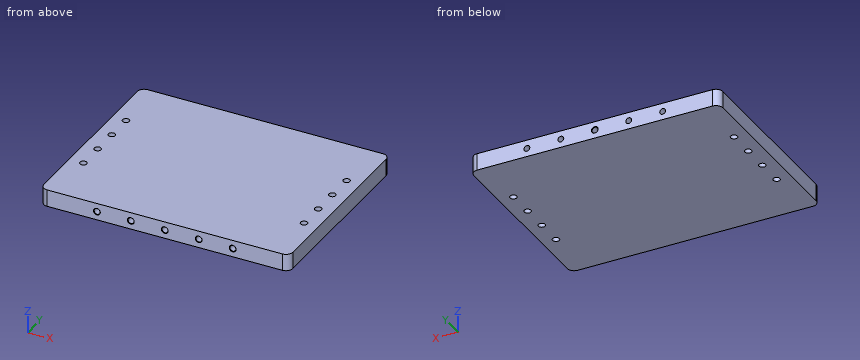
from build123d import *

# Parameters (mm, degrees)
SKETCH_1_R          = 1.5
EXTRUDE_1_DEPTH     = 7.5
SKETCH_2_R          = 1.3
CUT_EXTRUDE_1_DEPTH = 7.5
CUT_EXTRUDE_START   = -7.5
SKETCH_3_R          = 1.3
CUT_EXTRUDE_2_DEPTH = 7.5
CHAMFER_1_SIZE      = 0.2
CHAMFER_2_SIZE      = 0.2


with BuildPart() as part:
    # Sketch 1 → Extrude 1 (new body)
    with BuildSketch(Plane.XY):
        with BuildLine():
            Line((-52, -42.5), (52, -42.5))
            ThreePointArc((52, -42.5), (54.121320344, -41.621320344), (55, -39.5))
            Line((55, -39.5), (55, 39.5))
            ThreePointArc((55, 39.5), (54.121320344, 41.621320344), (52, 42.5))
            Line((52, 42.5), (-52, 42.5))
            ThreePointArc((-52, 42.5), (-54.121320344, 41.621320344), (-55, 39.5))
            Line((-55, 39.5), (-55, -39.5))
            ThreePointArc((-55, -39.5), (-54.121320344, -41.621320344), (-52, -42.5))
        make_face()
        with Locations((48.75, 18)):
            Circle(SKETCH_1_R, mode=Mode.SUBTRACT)
        with Locations((48.75, 6)):
            Circle(SKETCH_1_R, mode=Mode.SUBTRACT)
        with Locations((48.75, -6)):
            Circle(SKETCH_1_R, mode=Mode.SUBTRACT)
        with Locations((48.75, -18)):
            Circle(SKETCH_1_R, mode=Mode.SUBTRACT)
        with Locations((-48.75, -18)):
            Circle(SKETCH_1_R, mode=Mode.SUBTRACT)
        with Locations((-48.75, -6)):
            Circle(SKETCH_1_R, mode=Mode.SUBTRACT)
        with Locations((-48.75, 6)):
            Circle(SKETCH_1_R, mode=Mode.SUBTRACT)
        with Locations((-48.75, 18)):
            Circle(SKETCH_1_R, mode=Mode.SUBTRACT)
    extrude(amount=EXTRUDE_1_DEPTH)

    # Sketch 2 → Cut-Extrude 1 (cut)
    with BuildSketch(Plane(origin=(0, 42.5, 0), x_dir=(1, 0, 0), z_dir=(0, 1, 0))):
        with Locations(Location((-15, -3.75, 0), (0, 0, 270))):
            Circle(SKETCH_2_R)
        with Locations(Location((30, -3.75, 0), (0, 0, 270))):
            Circle(SKETCH_2_R)
        with Locations(Location((0, -3.75, 0), (0, 0, 270))):
            Circle(SKETCH_2_R)
        with Locations(Location((15, -3.75, 0), (0, 0, 270))):
            Circle(SKETCH_2_R)
        with Locations(Location((-30, -3.75, 0), (0, 0, 270))):
            Circle(SKETCH_2_R)
    extrude(amount=-CUT_EXTRUDE_1_DEPTH, mode=Mode.SUBTRACT)

    # Sketch 3 → Cut-Extrude 2 (cut)
    with BuildSketch(Plane(origin=(0, -42.5, 0), x_dir=(-1, 0, 0), z_dir=(0, -1, 0)).offset(CUT_EXTRUDE_START)):
        with Locations(Location((-15, -3.75, 0), (0, 0, 270))):
            Circle(SKETCH_3_R)
        with Locations(Location((-30, -3.75, 0), (0, 0, 270))):
            Circle(SKETCH_3_R)
        with Locations(Location((0, -3.75, 0), (0, 0, 270))):
            Circle(SKETCH_3_R)
        with Locations(Location((15, -3.75, 0), (0, 0, 270))):
            Circle(SKETCH_3_R)
        with Locations(Location((30, -3.75, 0), (0, 0, 270))):
            Circle(SKETCH_3_R)
    extrude(amount=CUT_EXTRUDE_2_DEPTH, mode=Mode.SUBTRACT)

    # Chamfer 1
    chamfer_1_edges = [part.edges().sort_by_distance(p)[0] for p in [
        (-30, 35, 2.45),
        (-15, 35, 2.45),
        (30, 35, 2.45),
        (15, 35, 2.45),
        (0, 42.5, 2.45),
    ]]
    chamfer(chamfer_1_edges, length=CHAMFER_1_SIZE)

    # Chamfer 2
    chamfer_2_edges = [part.edges().sort_by_distance(p)[0] for p in [
        (-30, -42.5, 2.45),
        (-15, -42.5, 2.45),
        (0, -42.5, 2.45),
        (30, -42.5, 2.45),
        (15, -42.5, 2.45),
    ]]
    chamfer(chamfer_2_edges, length=CHAMFER_2_SIZE)


solid = part.part
Geometry: final body of the model. Coordinates: model frame, mm. Coordinates: 2 decimals unless noted, no trailing zeros. Order: outer loops, then holes, each group sorted by start corner. A loop starts at its lowest first (then second) coordinate and runs counter-clockwise, first axis right, second up.
(1) Section query B-B (y = -6). Return the cut outline in (x, z), plus the area to 3 significant figures.
(2) Section query A-A (x = -48.75). Return the cut outline in (y, z), plus the area to 4 significant figures.
(3) Section query C-C (x = 0). Return the cut outline in (y, z), plus the area to 3 significant figures.
(4) First-contact query: pin 1 (1.8 mm diameter, centred on x = 15, z = 3.5, fed in from +Y); pin 2 (2 mm diameter, centred on x = 0, z = 3.75, fed in from +Y); pin 3 (0.8 mm diameter, centred on x = -29.5, z = 3.5, fed in from -Y). Flat tips, straight axial feed; report the tip coordinate or a pass-through.
(5) Material intervals for probe 1 along Y at (x, z) = (48.5, 7); probe 2 along X at (y, z) = (39, 3); probe 3 along Z at (x, y) = (15, -36.25), sorted ascending.
Solution:
1. outline: (-55, 0) - (-50.25, 0) - (-50.25, 7.5) - (-55, 7.5) - close; (-47.25, 0) - (47.25, 0) - (47.25, 7.5) - (-47.25, 7.5) - close; (50.25, 0) - (55, 0) - (55, 7.5) - (50.25, 7.5) - close
1. area: 780 mm2
2. outline: (-42.5, 0) - (-19.5, 0) - (-19.5, 7.5) - (-42.5, 7.5) - close; (-16.5, 0) - (-7.5, 0) - (-7.5, 7.5) - (-16.5, 7.5) - close; (-4.5, 0) - (4.5, 0) - (4.5, 7.5) - (-4.5, 7.5) - close; (7.5, 0) - (16.5, 0) - (16.5, 7.5) - (7.5, 7.5) - close; (19.5, 0) - (42.5, 0) - (42.5, 7.5) - (19.5, 7.5) - close
2. area: 547.5 mm2
3. outline: (-42.5, 0) - (42.5, 0) - (42.5, 2.25) - (42.3, 2.45) - (35, 2.45) - (35, 5.05) - (42.3, 5.05) - (42.5, 5.25) - (42.5, 7.5) - (-42.5, 7.5) - (-42.5, 5.25) - (-42.3, 5.05) - (-35, 5.05) - (-35, 2.45) - (-42.3, 2.45) - (-42.5, 2.25) - close
3. area: 598 mm2
4. pin 1: stops at y = 35.05
4. pin 2: stops at y = 35
4. pin 3: stops at y = -35
5. probe 1: y = -42.5 to -19.48, -16.52 to -7.48, -4.52 to 4.52, 7.48 to 16.52, 19.48 to 42.5
5. probe 2: x = -55 to -31.06, -28.94 to -16.06, -13.94 to -1.06, 1.06 to 13.94, 16.06 to 28.94, 31.06 to 55
5. probe 3: z = 0 to 2.45, 5.05 to 7.5
